Input: part model. Units: mm. Frame: model coordinates. A direction names the side the tool comes from. Coordinates: 2 decimals unless noted, no trailing zeros. Loops run counter-clockwise (first coordinate to the right, second up) from the corner with the lowest first, then second, coordinate; pieces in that order, holes last. Notation, with made-up numbers: (57.25, 58.25) - (66.25, 58.25) arc R15 cw to (66.25, 72.25) - close; hole circle Ø8 at (55.5, -12.75). An arc over 180 degrees is marked (long way). Answer as CSV lines item,"result". Start each with the question number.
```python
from build123d import *

# Parameters (mm, degrees)
BLANKSKE_W          = 100
BLANKSKE_H          = 6
BLANK_DEPTH         = 10
TOOTHCUTSIM_DEPTH   = 101.677703589
TEETHCUTS_COUNT     = 33
TEETHCUTS_PITCH     = 3.14159265
SKETCH_1_W          = 19.29399127
SKETCH_1_H          = 9.471097972
CUT_EXTRUDE_1_DEPTH = 10
SKETCH_2_W          = 10
SKETCH_2_H          = 3.75
EXTRUDE_1_DEPTH     = 10
SKETCH_3_R          = 1.6
CUT_EXTRUDE_2_DEPTH = 10
CUT_EXTRUDE_3_DEPTH = 2


with BuildPart() as part:
    # BlankSke → Blank (new body)
    with BuildSketch(Plane.XY):
        with Locations((50, 3)):
            Rectangle(BLANKSKE_W, BLANKSKE_H)
    extrude(amount=-BLANK_DEPTH)

    # TooCutSkeSim → ToothCutSim (cut, through all)
    with BuildSketch(Plane.XY):
        Polygon((0.44443537, 3.75), (-0.44443537, 3.75), (-1.272613241, 6.0254), (1.272613241, 6.0254), align=None)
    toothcutsim = extrude(amount=-TOOTHCUTSIM_DEPTH, mode=Mode.SUBTRACT)

    # TeethCuts: ToothCutSim ×33
    with Locations(*[(i * TEETHCUTS_PITCH, 0, 0) for i in range(1, TEETHCUTS_COUNT)]):
        add(toothcutsim, mode=Mode.SUBTRACT)

    # Sketch 1 → Cut-Extrude 1 (cut)
    with BuildSketch(Plane.XY):
        with Locations((9.646995635, 8.485548986)):
            Rectangle(SKETCH_1_W, SKETCH_1_H)
    extrude(amount=-CUT_EXTRUDE_1_DEPTH, mode=Mode.SUBTRACT)

    # Sketch 2 → Extrude 1 (add)
    with BuildSketch(Plane.ZY):
        with Locations((-5, 1.875)):
            Rectangle(SKETCH_2_W, SKETCH_2_H)
    extrude(amount=EXTRUDE_1_DEPTH)

    # Sketch 3 → Cut-Extrude 2 (cut)
    with BuildSketch(Plane(origin=(0, 3.75, 0), x_dir=(1, 0, 0), z_dir=(0, 1, 0))):
        with Locations(Location((0, 5, 0), (0, 0, 270))):
            Circle(SKETCH_3_R)
        with Locations(Location((10, 5, 0), (0, 0, 270))):
            Circle(SKETCH_3_R)
    extrude(amount=-CUT_EXTRUDE_2_DEPTH, mode=Mode.SUBTRACT)

    # Sketch 4 → Cut-Extrude 3 (cut)
    with BuildSketch(Plane(origin=(0, 3.75, 0), x_dir=(1, 0, 0), z_dir=(0, 1, 0))):
        Polygon((-1.58771324, 7.75), (-3.175426481, 5), (-1.58771324, 2.25), (1.58771324, 2.25), (3.175426481, 5), (1.58771324, 7.75), align=None)
        Polygon((8.41228676, 7.75), (6.824573519, 5), (8.41228676, 2.25), (11.58771324, 2.25), (13.175426481, 5), (11.58771324, 7.75), align=None)
    extrude(amount=-CUT_EXTRUDE_3_DEPTH, mode=Mode.SUBTRACT)


solid = part.part
```
Item 1: Set-up query: faces 1 (the flat face through (46.276, 4.859, -4.93)), 2 (the flat face through (0, 3, -2.25)), 3 (the flat face through (19.71, 4.89, -4.93)). Return all of +Z, -Z, +X, -X, +Y, -Y with unobstructed straight access to the full face (end or side cutting, diameter ignored); none if empty.
Item 2: Draft query along Z for faces 4 (the flat face through (12.37, 2.764, -3.606)), 5 (the flat face through (47.984, 4.891, -4.93)). Return one class per face: pulls with the +Z half, pulls with the -Z half, needs draft (parallel to the pull), parting line crosses it, or undercut.
Item 3: Material intervals for probe 1 along X at (y, z) = (0.4, -5); probe 2 along X at (y, z) = (3.25, -3); probe 3 along Y at (x, z) = (59.5, -6), sorted ascending.
Item 4: Contact query for a flat-ended pin moving along its axis: P1, Ø4.5, axis at x = 9.5, z = -4.5, coming from the +Y side. Output: stop coordinate, or through.
Item 5: Section query A-A, the plane x = 10. Output: boundary loops of the cut face in (y, z).
Response values:
1,face 1,"+Z, -Z, +Y"
1,face 2,"+Y"
1,face 3,"+Z, -Z, -X, +Y"
2,face 4,"undercut"
2,face 5,"needs draft"
3,probe 1,"x = -10 to -1.6, 1.6 to 8.4, 11.6 to 100"
3,probe 2,"x = -10 to -2.02, 2.02 to 7.98, 12.02 to 100"
3,probe 3,"y = 0 to 3.75"
4,P1,"stops at y = 3.75"
5,outline,"(0, -10) - (3.75, -10) - (3.75, -7.75) - (1.75, -7.75) - (1.75, -6.6) - (0, -6.6) - close; (0, -3.4) - (1.75, -3.4) - (1.75, -2.25) - (3.75, -2.25) - (3.75, 0) - (0, 0) - close"
